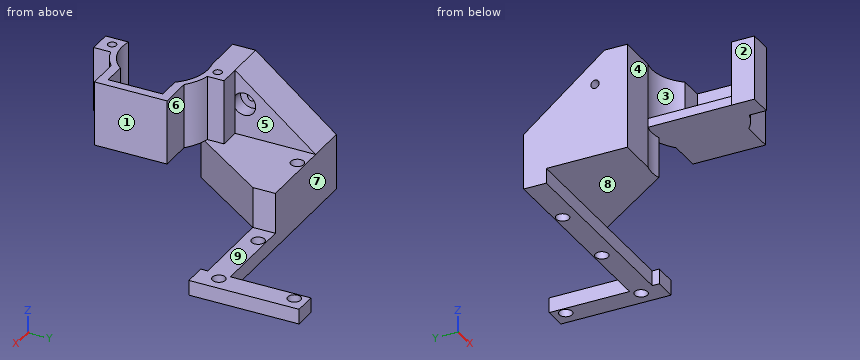
Autodesk Inventor part; units mm, degrees
ref_plane "Work Plane3" through (-42.5, -74.75, 21.5715) normal (0, 0, -1) x (0, 1, 0)
ref_plane "YZ Plane" through (0, 0, 0) normal (1, 0, 0) x (0, 1, 0)
ref_plane "XZ Plane" through (0, 0, 0) normal (0, 1, 0) x (-1, 0, 0)
ref_plane "Work Plane1" through (0, 0, 0) normal (0, 0, 1) x (1, 0, 0)
sketch "Sketch1" plane through (0, 0, 0) normal (0, 0, 1) x (1, 0, 0)
  line L0 (-45, 22) -> (22, 22)
  line L1 (22, 22) -> (22, -22)
  line L2 (22, -22) -> (-45, -22)
  line L3 (-45, -28) -> (-45, -22)
  line L4 (-30, -28) -> (-45, -28)
  line L5 (-30, -28) -> (-28, -30)
  line L6 (-28, -30) -> (28, -30)
  line L7 (28, -30) -> (30, -28)
  line L8 (30, -28) -> (30, 28)
  line L9 (30, 28) -> (28, 30)
  line L10 (28, 30) -> (-28, 30)
  line L11 (-28, 30) -> (-30, 28)
  line L12 (-30, 28) -> (-45, 28)
  line L13 (-45, 22) -> (-45, 28)
  circle A0 centre (25, 25) radius 1.95
  circle A1 centre (25, 0) radius 1.95
  circle A2 centre (0, 25) radius 1.95
  circle A3 centre (-25, -25) radius 1.95
  circle A4 centre (25, -25) radius 1.95
  circle A5 centre (-25, 25) radius 1.95
  circle A6 centre (0, -25) radius 1.95
  line L14 (30, 4.1832) -> (22.5, 4.1832)
  line L15 (22.5, 4.1832) -> (22.5, -32.3594)
  line L16 (22.5, -32.3594) -> (30, -32.3594)
  line L17 (30, -32.3594) -> (30, 4.1832)
  line L18 (22.5, -22.5) -> (-45, -22.5)
  line L19 (-45, -22.5) -> (-45, -30)
  line L20 (-45, -30) -> (22.5, -30)
  line L21 (22.5, -30) -> (22.5, -22.5)
  circle A7 centre (25, 0) radius 2.15
  circle A8 centre (25, -25) radius 2.15
  circle A9 centre (0, -25) radius 2.15
  circle A10 centre (-25, -25) radius 2.15
  point P0 (0, 0)
  dimension "d0" = 0
  dimension "d1" = 0.5
  dimension "d2" = 0.5
  dimension "d3" = 0.2
  dimension "d4" = 0.2
  dimension "d5" = 0.2
  dimension "d6" = 0.2
extrude "Extrusion1" add sketch "Sketch1" along normal blind 5 contours L18 L15 L6 L5 L4 L3 | L4 L5 L20 L19 | L15 L14 L8 L7 L6 | L6 L7 L17 L16 L15
ref_plane "Work Plane2" through (-32, -78.0277, 40.0715) normal (0, 0, -1) x (0, 1, 0)
sketch "Sketch2" plane through (-32, -78.0277, 40.0715) normal (0, 0, -1) x (0, 1, 0)
  arc A0 (-8.1223, 3.5) -> (-12.3223, 3.5) centre (-10.2223, 3.5) ccw
  arc A1 (-1.4723, 14.4287) -> (-6.2777, 7) centre (7.2777, 3.5) ccw
  arc A2 (20.8332, 7) -> (16.0277, 14.4287) centre (7.2777, 3.5) ccw
  arc A3 (22.6777, 3.5) -> (26.8777, 3.5) centre (24.7777, 3.5) ccw
  line L0 (-6.2777, 0) -> (-10.2223, 0)
  arc A4 (-6.7223, 3.5) -> (21.2777, 3.5) centre (7.2777, 3.5) ccw
  line L1 (-6.5873, 0) -> (-14.2223, 0)
  line L2 (-14.2223, 0) -> (-14.2223, 7.5835)
  line L3 (-14.2223, 7.5835) -> (-8.5689, 7.5835)
  line L4 (21.1796, 0.1492) -> (27.0132, 0.1492)
  line L5 (27.0132, 0.1492) -> (28.7777, 0.1492)
  line L6 (28.7777, 0.1492) -> (28.7777, 7.1168)
  line L7 (28.7777, 7.1168) -> (23.2373, 7.1168)
  circle A5 centre (24.7777, 3.5) radius 1.4
  circle A6 centre (-10.2223, 3.5) radius 1.4
  line L8 (-1.7723, 14.5719) -> (-4.7723, 14.5719)
  line L9 (-4.7723, 14.5719) -> (-4.7723, 25.3)
  line L10 (-4.7723, 25.3) -> (-1.7723, 25.3)
  line L11 (-1.7723, 25.3) -> (-1.7723, 14.5719)
  line L12 (16.3277, 14.5719) -> (19.3277, 14.5719)
  line L13 (19.3277, 14.5719) -> (19.3277, 25.3)
  line L14 (19.3277, 25.3) -> (16.3277, 25.3)
  line L15 (16.3277, 25.3) -> (16.3277, 14.5719)
  line L16 (16.3277, 25.3) -> (-1.7723, 25.3)
  line L17 (-1.7723, 25.3) -> (-1.7723, 22.3)
  line L18 (-1.7723, 22.3) -> (16.3277, 22.3)
  line L19 (16.3277, 22.3) -> (16.3277, 25.3)
  arc A7 (21.1796, 0.1492) -> (16.3277, 14.5719) centre (7.2777, 3.5) ccw
  arc A8 (-1.7723, 14.5719) -> (-6.5873, 0) centre (7.2777, 3.5) ccw
  arc A9 (23.2373, 7.1168) -> (19.3277, 14.5719) centre (7.2777, 3.5) ccw
  arc A10 (-4.7723, 14.5719) -> (-8.5689, 7.5835) centre (7.2777, 3.5) ccw
  line L20 (-1.4723, 22) -> (16.0277, 22)
  point P0 (78.0277, 32)
  dimension "d14" = 2.8
  dimension "d15" = 2.8
  dimension "d16" = 4
  dimension "d17" = 4
  dimension "d33" = 3
  dimension "d36" = 3
  dimension "d37" = 3
  dimension "d40" = 0.3
  dimension "d41" = 0.3
  dimension "d42" = 0.3
  dimension "d43" = 0.3
  dimension "d44" = 0.3
ref_plane "Work Plane3" through (-42.5, -74.75, 21.5715) normal (0, 0, -1) x (0, 1, 0)
extrude "Extrusion2" add sketch "Sketch2" along normal up to surface (18.5 mm away)
sketch "Sketch3" plane through (-24.8832, -49.25, 21.5715) normal (0, 0, -1) x (-1, 0, 0)
  arc A0 (6.9676, -7.5981) -> (-7.4551, -12.45) centre (3.6168, -21.5) ccw
  line L0 (6.9676, 0) -> (6.9676, -7.5981)
  line L1 (0, 0) -> (6.9676, 0)
  line L2 (0, -5.5404) -> (0, 0)
  arc A1 (0, -5.5404) -> (-7.4551, -9.45) centre (3.6168, -21.5) ccw
  circle A2 centre (3.6168, -4) radius 1.4
  arc A3 (6.9676, -7.5981) -> (-7.4551, -12.45) centre (3.6168, -21.5) ccw
  line L3 (-18.1832, -9.45) -> (-7.4551, -9.45)
  line L4 (-15.1832, -12.45) -> (-15.1832, -30.55)
  line L5 (-7.4551, -12.45) -> (-15.1832, -12.45)
  line L6 (-18.1832, -33.55) -> (-18.1832, -9.45)
  line L7 (-7.4551, -33.55) -> (-18.1832, -33.55)
  arc A4 (-7.4551, -33.55) -> (-0.4667, -37.3466) centre (3.6168, -21.5) ccw
  line L8 (-0.4667, -43) -> (-0.4667, -37.3466)
  line L9 (7.1168, -43) -> (-0.4667, -43)
  line L10 (7.1168, -35.3651) -> (7.1168, -43)
  arc A5 (-7.4551, -30.55) -> (7.1168, -35.3651) centre (3.6168, -21.5) ccw
  line L11 (-15.1832, -30.55) -> (-7.4551, -30.55)
  line L12 (7.1168, -35.3651) -> (6.9676, -7.5981)
  point P0 (-24.8832, 49.25)
  point P1 (7.3934, -35.5712)
extrude "Extrusion3" add sketch "Sketch3" along normal blind 3 contours L12 A5 L11 L4 L5 A0 | A0 L5 L4 L11 A5 L10 L9 L8 A4 L7 L6 L3 A1 L2 L1 L0 | A2
sketch "Sketch4" plane through (0, 0, 5) normal (0, 0, 1) x (1, 0, 0)
  circle A0 centre (25, 0) radius 2.15
  circle A1 centre (25, -25) radius 2.15
  circle A2 centre (-25, -25) radius 2.15
  circle A3 centre (0, -25) radius 2.15
  line L0 (22.5, -22.5) -> (-45, -22.5)
  line L1 (-45, -22.5) -> (-45, -30)
  line L2 (-45, -30) -> (22.5, -30)
  line L3 (22.5, -30) -> (22.5, -32.3594)
  line L4 (22.5, -32.3594) -> (30, -32.3594)
  line L5 (30, -32.3594) -> (30, 4.1832)
  line L6 (30, 4.1832) -> (22.5, 4.1832)
  line L7 (22.5, 4.1832) -> (22.5, -22.5)
  arc A4 (-25, -57.1946) -> (-32, -57.1946) centre (-28.5, -70.75) ccw
  line L8 (-45, -22.5) -> (-45, -30)
  arc A5 (-17.4281, -61.7) -> (-31.8508, -56.8481) centre (-28.5, -70.75) ccw
  line L9 (-45, -22.5) -> (-31.8508, -22.5)
  line L10 (-31.8508, -22.5) -> (-31.8508, -56.8481)
  line L11 (-31.8508, -56.8481) -> (-45, -56.8481)
  line L12 (-45, -56.8481) -> (-45, -22.5)
  line L13 (-25, -56.8849) -> (-6.175, -30)
  line L14 (-45, -30) -> (22.5, -30)
  line L15 (-25, -56.8849) -> (7.8204, -56.8849) construction
  line L16 (-6.175, -30) -> (-6.175, -22.5)
  line L17 (22.5, -22.5) -> (-45, -22.5)
  line L18 (-25, -53.25) -> (-25, -57.1946)
  line L19 (-31.8508, -22.5) -> (-6.175, -22.5)
  line L20 (-6.175, -22.5) -> (-6.175, -30)
  line L21 (-6.175, -30) -> (-31.8508, -30)
  line L22 (-31.8508, -30) -> (-31.8508, -22.5)
  point P0 (0, 0)
  point P1 (-32, -84.6151)
  dimension "d20" = 55
extrude "Extrusion4" add sketch "Sketch4" along normal up to surface (13.5715 mm away) contours L16 L2 L10 L0 | L10 L2 L1 L0 | L13 A5 L10 L2 | L10 L11 L12 L2
sketch "Sketch5" plane through (-45, -30, 0) normal (-1, 0, 0) x (0, 0, 1)
  line L0 (40.0715, -26.8481) -> (40.0715, -19.25)
  line L1 (40.0715, -19.25) -> (18.5715, -19.25)
  line L2 (18.5715, -26.8481) -> (18.5715, 7.5)
  line L3 (40.0715, -26.8481) -> (40.0715, -19.25)
  line L4 (0, 7.5) -> (18.5715, 7.5)
  line L5 (40.0715, -19.25) -> (18.5715, 7.5)
  line L6 (40.0715, -26.8481) -> (21.5715, -26.8481)
  line L7 (21.5715, -26.8481) -> (18.5715, -26.8481)
  line L8 (18.5715, -26.8481) -> (18.5715, -19.25)
  line L9 (40.0715, -19.25) -> (18.5715, -19.25)
  line L10 (18.5715, -19.25) -> (18.5715, 7.5)
  line L11 (18.5715, 7.5) -> (40.0715, -19.25)
  line L12 (40.0715, -19.25) -> (18.5715, -19.25)
  line L13 (18.5715, -19.25) -> (18.5715, -26.8481)
  line L14 (18.5715, -26.8481) -> (40.0715, -26.8481)
  line L15 (40.0715, -26.8481) -> (40.0715, -19.25)
  point P0 (0, 30)
  point P1 (5, 7.5)
extrude "Extrusion5" add sketch "Sketch5" against normal up to surface (13.1492 mm away)
sketch "Sketch6" plane through (-31.8508, -49.25, 18.5715) normal (1, 0, 0) x (0, 0, -1)
  line L0 (-21.5, 0) -> (0, 0)
  line L1 (0, 26.75) -> (0, 0)
  circle A0 centre (-10.75, 3.0956) radius 1.4
  line L2 (0, 26.75) -> (-21.5, 0)
  point P0 (18.5715, 49.25)
  dimension "d25" = 2.8
hole "Hole1" at (-31.8508, -46.1544, 29.3215) direction (-1, 0, 0) diameter 2.8 depth 20 tip angle 118 counterbore diameter 7.5 counterbore depth 4.775
properties part number "cellSTORM_v5_focusmotormount"
Can you work these out from the model? Positions are in its coordinate system, mm. Face numbers are marked on the shaded views. A direction names the side the tool comes from. Coordinates: 2 decimals unless noted, no trailing zeros. Order: outer loops, then holes, each group sorted by start corner. A loop starts at its lowest first (then second) coordinate and runs counter-clockwise, first axis right, second up. Notation, with made-up numbers: (25.25, -28.75) -> (61.25, -28.75) arc R30 ccw to (61.25, -0.75) -> close; hole circle Ø10 at (63, 16). An arc over 180 degrees is marked (long way). Use one line per item in the form item = value.
Q1. Imagine slicing it at D-D, the plane y = -88.25. List the corners of the cut face in (x, z) for me.
From the geometry:
outline = (-32, 18.57) -> (-24.42, 18.57) -> (-24.42, 40.07) -> (-27.1, 40.07) -> (-27.1, 21.57) -> (-29.9, 21.57) -> (-29.9, 40.07) -> (-32, 40.07) -> close
Q2. I need wall thicknesses on L1, parallel to Y at x = 25, z = 2.9; L2, parallel to X at y = -88.25, z = 31.5; L3, parallel to Y at x = 0, z = 2. Which ranges of each line are inside material? Lowest first, please.
From the geometry:
L1 = -32.36 to -27.15, -22.85 to -2.15, 2.15 to 4.18
L2 = -32 to -29.9, -27.1 to -24.42
L3 = -30 to -27.15, -22.85 to -22.5
Q3. Imagine slicing it at B-B, the plane x = 25. List the corners of the cut face in (y, z) for me, then the cut area to 3 significant figures.
From the geometry:
outline = (-32.36, 0) -> (-27.15, 0) -> (-27.15, 5) -> (-32.36, 5) -> close; (-22.85, 0) -> (-2.15, 0) -> (-2.15, 5) -> (-22.85, 5) -> close; (2.15, 0) -> (4.18, 0) -> (4.18, 5) -> (2.15, 5) -> close
area = 140 mm²
Q4. Which directions (+Z, -Z, +X, -X, +Y, -Y) give clear straight access to the entire face, cutting with the end or side of a thin tool? Please do the marked faces 5, 6, 7, 8 and 9.
From the geometry:
face_5 = +Z, +X, +Y
face_6 = +Z, -Z, +X, +Y
face_7 = +Z, -Z, -X, +Y
face_8 = -Z, -X, -Y
face_9 = +Z, +X, +Y, -Y
Q5. Imagine slicing it at A-A, the plane y = 0. List the corners of the cut face in (x, z) for me.
From the geometry:
outline = (22.5, 0) -> (22.85, 0) -> (22.85, 5) -> (22.5, 5) -> close; (27.15, 0) -> (30, 0) -> (30, 5) -> (27.15, 5) -> close
Q6. Imagine slicing it at C-C, the plane z = 36. Give the number of separate pieces and of enclosed holes in the cut face, then the cut area to 3 significant figures.
From the geometry:
separate_pieces = 1
enclosed_holes = 2
area = 415 mm²
Q7. Will these pins go through, and if not, where does the flat tip stop? P1, Ø7, axis at x = 25, y = -25, coming from the +Z side; P2, Ø4, axis at y = -68.5, z = 30, coming from the +X side; P3, Ø2, axis at y = -26, z = 11, coming from the +X side (3 decimals).
From the geometry:
P1 = 5
P2 = -6.7
P3 = -6.175
Q8. We'd pull the mould along X, two halves only. Please class the marked faces 1, 2, 3 and 4: released by +X, released by -X, zero draft, split by the parting line, or undercut.
From the geometry:
face_1 = released by +X
face_2 = released by -X
face_3 = undercut
face_4 = zero draft
